```python
from build123d import *

# Parameters (mm, degrees)
CYLINDER078_R     = 1.5
CYLINDER078_DEPTH = 10
BOX015_W          = 5.75
BOX015_H          = 2.75
BOX015_DEPTH      = 10
BOX014_W          = 2.75
BOX014_H          = 34
BOX014_DEPTH      = 10
BOX013_W          = 5.75
BOX013_H          = 2.75
BOX013_DEPTH      = 10
BOX012_W          = 2.75
BOX012_H          = 34
BOX012_DEPTH      = 10
CYLINDER077_R     = 1.5
CYLINDER077_DEPTH = 10
BOX011_W          = 17.5
BOX011_H          = 21
BOX011_DEPTH      = 1.01
BOX009_W          = 20
BOX009_H          = 20
BOX009_DEPTH      = 1.01
BOX008_W          = 20
BOX008_H          = 20
BOX008_DEPTH      = 1.01
BOX007_W          = 20
BOX007_H          = 70
BOX007_DEPTH      = 1.01
BOX010_W          = 17.5
BOX010_H          = 21
BOX010_DEPTH      = 1.01


with BuildPart() as shieldcrosshole1:
    # Cylinder078 → Cylinder078 (new body)
    with BuildSketch(Plane(origin=(105, 116, 34), x_dir=(1, 0, 0), z_dir=(0, 0, 1))):
        Circle(CYLINDER078_R)
    extrude(amount=CYLINDER078_DEPTH)


with BuildPart() as cube007:
    # Box015 → Box015 (new body)
    with BuildSketch(Plane(origin=(115, 146.625, 34), x_dir=(1, 0, 0), z_dir=(0, 0, 1))):
        with Locations((2.875, 1.375)):
            Rectangle(BOX015_W, BOX015_H)
    extrude(amount=BOX015_DEPTH)


with BuildPart() as cube006:
    # Box014 → Box014 (new body)
    with BuildSketch(Plane(origin=(115, 146.75, 34), x_dir=(1, 0, 0), z_dir=(0, 0, 1))):
        with Locations((1.375, 17)):
            Rectangle(BOX014_W, BOX014_H)
    extrude(amount=BOX014_DEPTH)


with BuildPart() as cube005:
    # Box013 → Box013 (new body)
    with BuildSketch(Plane(origin=(89.25, 146.625, 34), x_dir=(1, 0, 0), z_dir=(0, 0, 1))):
        with Locations((2.875, 1.375)):
            Rectangle(BOX013_W, BOX013_H)
    extrude(amount=BOX013_DEPTH)


with BuildPart() as cube004:
    # Box012 → Box012 (new body)
    with BuildSketch(Plane(origin=(92.25, 146.75, 34), x_dir=(1, 0, 0), z_dir=(0, 0, 1))):
        with Locations((1.375, 17)):
            Rectangle(BOX012_W, BOX012_H)
    extrude(amount=BOX012_DEPTH)


with BuildPart() as shieldcuts:
    # Cylinder077 → Cylinder077 (new body)
    with BuildSketch(Plane(origin=(105, 175, 34), x_dir=(1, 0, 0), z_dir=(0, 0, 1))):
        Circle(CYLINDER077_R)
    extrude(amount=CYLINDER077_DEPTH)

    # Fusion037: union ShieldCrossHole1, Cube007, Cube006, Cube005, Cube004
    add(shieldcrosshole1.part)
    add(cube007.part)
    add(cube006.part)
    add(cube005.part)
    add(cube004.part)


with BuildPart() as shieldcross007:
    # Box011 → Box011 (new body)
    with BuildSketch(Plane(origin=(117.5, 117, 39), x_dir=(1, 0, 0), z_dir=(0, 0, 1))):
        with Locations((8.75, 10.5)):
            Rectangle(BOX011_W, BOX011_H)
    extrude(amount=BOX011_DEPTH)


with BuildPart() as shieldcross005:
    # Box009 → Box009 (new body)
    with BuildSketch(Plane(origin=(75, 138, 39), x_dir=(1, 0, 0), z_dir=(0, 0, 1))):
        with Locations((10, 10)):
            Rectangle(BOX009_W, BOX009_H)
    extrude(amount=BOX009_DEPTH)


with BuildPart() as shieldcross004:
    # Box008 → Box008 (new body)
    with BuildSketch(Plane(origin=(115, 138, 39), x_dir=(1, 0, 0), z_dir=(0, 0, 1))):
        with Locations((10, 10)):
            Rectangle(BOX008_W, BOX008_H)
    extrude(amount=BOX008_DEPTH)


with BuildPart() as shieldcross003:
    # Box007 → Box007 (new body)
    with BuildSketch(Plane(origin=(95, 109.75, 39), x_dir=(1, 0, 0), z_dir=(0, 0, 1))):
        with Locations((10, 35)):
            Rectangle(BOX007_W, BOX007_H)
    extrude(amount=BOX007_DEPTH)


with BuildPart() as shieldfold:
    # Box010 → Box010 (new body)
    with BuildSketch(Plane(origin=(75, 158, 39), x_dir=(1, 0, 0), z_dir=(0, 0, 1))):
        with Locations((8.75, 10.5)):
            Rectangle(BOX010_W, BOX010_H)
    extrude(amount=BOX010_DEPTH)

    # Fusion036: union ShieldCross007, ShieldCross005, ShieldCross004, ShieldCross003
    add(shieldcross007.part)
    add(shieldcross005.part)
    add(shieldcross004.part)
    add(shieldcross003.part)

    # Cut009: cut ShieldCuts
    add(shieldcuts.part, mode=Mode.SUBTRACT)


solid = shieldfold.part
```
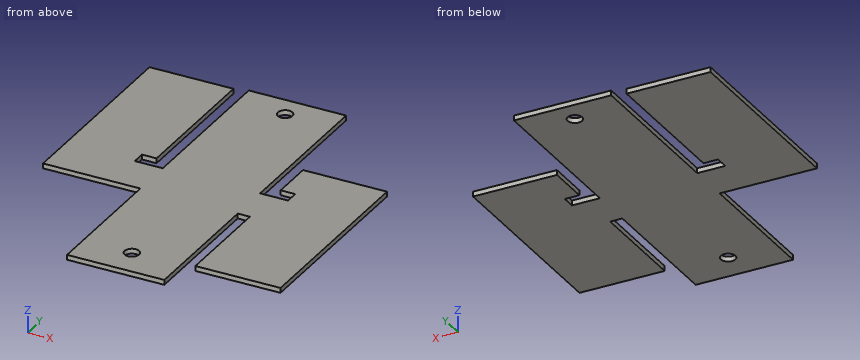
Geometry: final body of the model. Coordinates: model frame, mm. Round coordinates to 2 decimals unless told otherwise and drop trailing zeros. Loops run counter-clockwise (first coordinate to the right, second up) from the corner with the lowest first, then second, coordinate; pieces in that order, holes last. Notation, with made-up numbers: (-25.5, -1) -> (9.5, -1) arc R30 cw to (9.5, 34) -> close; hole circle Ø1 at (21.5, 55.25). An arc over 180 degrees is marked (long way). Use one line per item in the form item = value. Start each with the question number.
1) Section C-C on z = 39.7. Output: boundary loops of the cut face in (x, y) (3 decimals).
2) Section D-D on y = 175. Output: boundary loops of the cut face in (x, z), then the cut area to 3 significant figures.
3) Section A-A on y = 116. Output: boundary loops of the cut face in (x, z), then the cut area to 3 significant figures.
4) Line query: L1, parallel to X at y = 175, z = 39.8; L2, parallel to X at y = 150, z = 39.35; L3, parallel to Y at x = 105, z = 39.85. Output: solid intervals per line, ascending.
5) Section B-B on x = 105. Output: boundary loops of the cut face in (y, z), then the cut area to 3 significant figures.
6) First-contact query: P1, Ø0.5, axis at y = 168, z = 39.5, coming from the +X side; P2, Ø0.5, axis at y = 130, z = 39.5, coming from the -X side. Flat tips, straight axial feed; report the tip coordinate or a pass-through.
Response:
q1.outline = (75, 138) -> (95, 138) -> (95, 109.75) -> (115, 109.75) -> (115, 138) -> (117.5, 138) -> (117.5, 117) -> (135, 117) -> (135, 158) -> (117.75, 158) -> (117.75, 149.375) -> (120.75, 149.375) -> (120.75, 146.625) -> (115, 146.625) -> (115, 179.75) -> (95, 179.75) -> (95, 146.625) -> (89.25, 146.625) -> (89.25, 149.375) -> (92.25, 149.375) -> (92.25, 179) -> (75, 179) -> close; hole circle Ø3 at (105, 116); hole circle Ø3 at (105, 175)
q2.outline = (75, 39) -> (92.25, 39) -> (92.25, 40.01) -> (75, 40.01) -> close; (95, 39) -> (103.5, 39) -> (103.5, 40.01) -> (95, 40.01) -> close; (106.5, 39) -> (115, 39) -> (115, 40.01) -> (106.5, 40.01) -> close
q2.area = 34.6 mm^2
q3.outline = (95, 39) -> (103.5, 39) -> (103.5, 40.01) -> (95, 40.01) -> close; (106.5, 39) -> (115, 39) -> (115, 40.01) -> (106.5, 40.01) -> close
q3.area = 17.2 mm^2
q4.L1 = 75 to 92.25, 95 to 103.5, 106.5 to 115
q4.L2 = 75 to 92.25, 95 to 115, 117.75 to 135
q4.L3 = 109.75 to 114.5, 117.5 to 173.5, 176.5 to 179.75
q5.outline = (109.75, 39) -> (114.5, 39) -> (114.5, 40.01) -> (109.75, 40.01) -> close; (117.5, 39) -> (173.5, 39) -> (173.5, 40.01) -> (117.5, 40.01) -> close; (176.5, 39) -> (179.75, 39) -> (179.75, 40.01) -> (176.5, 40.01) -> close
q5.area = 64.6 mm^2
q6.P1 = 115
q6.P2 = 95
